Source: CAD feature listing. Evaluate the final solid. Frame: model axes, mm. Face numbers are marked on the shaded views. Coordinates: 2 decimals unless noted, no trailing zeros. Loops run counter-clockwise (first coordinate to the right, second up) from the corner with the lowest first, then second, coordinate; pieces in that order, holes last.
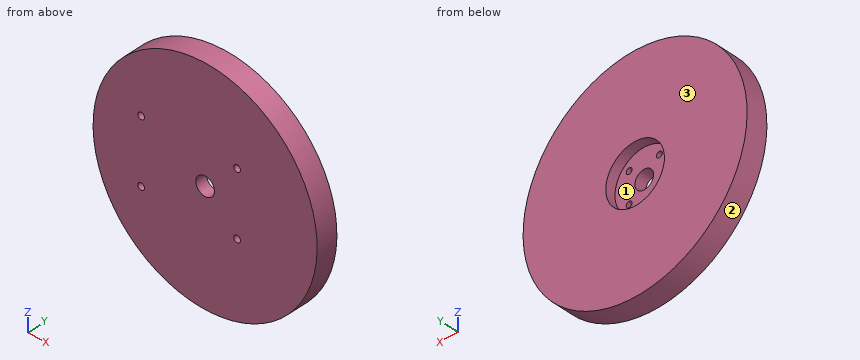
```python
from build123d import *

# Parameters (mm, degrees)
SCHIZZO1_R                   = 42
ESTRUSIONE_ESTRUSIONE1_DEPTH = 8
SCHIZZO2_R                   = 3.5
TAGLIO_ESTRUSIONE1_DEPTH     = 60.933296255
SCHIZZO4_R                   = 11
TAGLIO_ESTRUSIONE2_DEPTH     = 3.7
SCHIZZO5_R                   = 1.1
TAGLIO_ESTRUSIONE3_DEPTH     = 3
SCHIZZO6_R                   = 1.25
TAGLIO_ESTRUSIONE4_DEPTH     = 6


with BuildPart() as part:
    # Schizzo1 → Estrusione-Estrusione1 (new body)
    with BuildSketch(Plane(origin=(0, 0, 0), x_dir=(1, 0, 0), z_dir=(0, 1, 0))):
        with Locations(Location((0, 0, 0), (0, 0, 270))):
            Circle(SCHIZZO1_R)
    extrude(amount=ESTRUSIONE_ESTRUSIONE1_DEPTH)

    # Schizzo2 → Taglio-Estrusione1 (cut, through all)
    with BuildSketch(Plane.XZ):
        with Locations(Location((0, 0, 0), (0, 0, 270))):
            Circle(SCHIZZO2_R)
    extrude(amount=-TAGLIO_ESTRUSIONE1_DEPTH, mode=Mode.SUBTRACT)

    # Schizzo4 → Taglio-Estrusione2 (cut)
    with BuildSketch(Plane(origin=(0, 8, 0), x_dir=(1, 0, 0), z_dir=(0, 1, 0))):
        with Locations(Location((0, 0, 0), (0, 0, 270))):
            Circle(SCHIZZO4_R)
    extrude(amount=-TAGLIO_ESTRUSIONE2_DEPTH, mode=Mode.SUBTRACT)

    # Schizzo5 → Taglio-Estrusione3 (cut)
    with BuildSketch(Plane(origin=(0, 4.3, 0), x_dir=(1, 0, 0), z_dir=(0, 1, 0))):
        with Locations(Location((-5.66, 5.66, 0), (0, 0, 270))):
            Circle(SCHIZZO5_R)
        with Locations(Location((5.66, 5.66, 0), (0, 0, 270))):
            Circle(SCHIZZO5_R)
        with Locations(Location((5.66, -5.66, 0), (0, 0, 270))):
            Circle(SCHIZZO5_R)
        with Locations(Location((-5.66, -5.66, 0), (0, 0, 270))):
            Circle(SCHIZZO5_R)
    extrude(amount=-TAGLIO_ESTRUSIONE3_DEPTH, mode=Mode.SUBTRACT)

    # Schizzo6 → Taglio-Estrusione4 (cut)
    with BuildSketch(Plane.XZ):
        with Locations(Location((12, 12, 0), (0, 0, 270))):
            Circle(SCHIZZO6_R)
        with Locations(Location((12, -12, 0), (0, 0, 90))):
            Circle(SCHIZZO6_R)
        with Locations(Location((-24, 12, 0), (0, 0, 270))):
            Circle(SCHIZZO6_R)
        with Locations(Location((-24, -12, 0), (0, 0, 90))):
            Circle(SCHIZZO6_R)
    extrude(amount=-TAGLIO_ESTRUSIONE4_DEPTH, mode=Mode.SUBTRACT)


solid = part.part
```
Q1. Section query C-C on x = 12. Return the cut outline in (y, z).
Q2. Material intervals for line 1 along X through (y, z) = (3.3, 12); line 2 along X through (y, z) = (2, 6); line 3 along Z through (x, y) = (13, 2.25), sorted ascending.
Q3. Section query D-D on z = 12. Return the cut outline in (x, y).
Q4. Draft query along Z for the marked faces 1, 2 and 3. Return one class per face: released by +Z, released by -Z, zero draft, split by the parting line, or undercut.
Q5. Section query B-B on x = 1.5. Return the cut outline in (y, z), then the cut area to 3 significant figures.
Q6. Section query A-A on z = 0. Return the cut outline in (x, y).
Q7. First-contact query: pin 1 Ø0.7 at (x, z) = (-6, 6) entering from +Y; pin 2 Ø2.5 at (x, z) = (5.66, -5.66) entering from +Y; pin 3 Ø1.2 at (x, z) = (12, 12.5) entering from -Y; pin 4 Ø11 at (x, z) = (-4.5, 3.5) entering from +Y. Flat tips, straight axial feed; report the tip coordinate or a pass-through.
Resolved:
1. outline: (0, -40.25) - (8, -40.25) - (8, 40.25) - (0, 40.25) - (0, 13.25) - (6, 13.25) - (6, 10.75) - (0, 10.75) - (0, -10.75) - (6, -10.75) - (6, -13.25) - (0, -13.25) - close
2. line 1: x = -40.25 to -25.25, -22.75 to 10.75, 13.25 to 40.25
2. line 2: x = -41.57 to -6.71, -4.61 to 4.61, 6.71 to 41.57
2. line 3: z = -39.94 to -12.75, -11.25 to 11.25, 12.75 to 39.94
3. outline: (-40.25, 0) - (-25.25, 0) - (-25.25, 6) - (-22.75, 6) - (-22.75, 0) - (10.75, 0) - (10.75, 6) - (13.25, 6) - (13.25, 0) - (40.25, 0) - (40.25, 8) - (-40.25, 8) - close
4. face 1: undercut
4. face 2: split by the parting line
4. face 3: zero draft
5. outline: (0, -41.97) - (8, -41.97) - (8, -10.9) - (4.3, -10.9) - (4.3, -3.16) - (0, -3.16) - close; (0, 3.16) - (4.3, 3.16) - (4.3, 10.9) - (8, 10.9) - (8, 41.97) - (0, 41.97) - close
5. area: 564 mm2
6. outline: (-42, 0) - (-3.5, 0) - (-3.5, 4.3) - (-11, 4.3) - (-11, 8) - (-42, 8) - close; (3.5, 0) - (42, 0) - (42, 8) - (11, 8) - (11, 4.3) - (3.5, 4.3) - close
7. pin 1: stops at y = 1.3
7. pin 2: stops at y = 4.3
7. pin 3: stops at y = 6
7. pin 4: stops at y = 8
